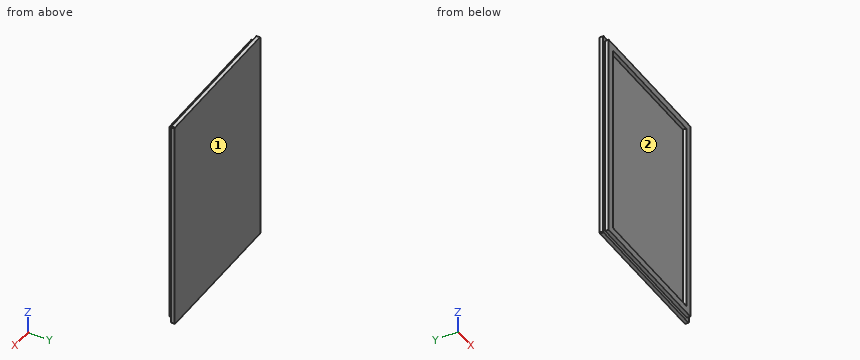
Autodesk Inventor part; units mm, degrees
ref_plane "YZ Plane" through (0, 0, 0) normal (1, 0, 0) x (0, 1, 0)
ref_plane "XZ Plane" through (0, 0, 0) normal (0, 1, 0) x (-1, 0, 0)
ref_plane "XY Plane" through (0, 0, 0) normal (0, 0, 1) x (1, 0, 0)
sketch "Sketch1" plane through (0, 0, 0) normal (0, 1, 0) x (-1, 0, 0)
  line L0 (0, 0) -> (210, 0)
  line L1 (210, 0) -> (210, -310)
  line L2 (210, -310) -> (0, -310)
  line L3 (0, -310) -> (0, 0)
  dimension "d0" = 310
  dimension "d1" = 210
extrude "Extrusion1" add sketch "Sketch1" along normal blind 5
chamfer "Chamfer1" distance 1 angle 45 4 edges at (0, 2.5, -310) (0, 2.5, 0) (-210, 2.5, -310) (-210, 2.5, 0)
sketch "Sketch2" plane through (0, 0, 0) normal (0, -1, 0) x (1, 0, 0)
  line L0 (-205, -305) -> (-5, -305)
  line L1 (-5, -305) -> (-5, -5)
  line L2 (-5, -5) -> (-205, -5)
  line L3 (-205, -5) -> (-205, -305)
  line L4 (0, -1) -> (0, -309)
  line L5 (-209, 0) -> (-1, 0)
  point P0 (0, 0)
  dimension "d7" = 300
  dimension "d8" = 200
  dimension "d9" = 5
  dimension "d10" = 5
extrude "Extrusion2" add sketch "Sketch2" along normal blind 5
sketch "Sketch3" plane through (0, -5, 0) normal (0, -1, 0) x (1, 0, 0)
  line L0 (-195, -295) -> (-15, -295)
  line L1 (-15, -295) -> (-15, -15)
  line L2 (-15, -15) -> (-195, -15)
  line L3 (-195, -15) -> (-195, -295)
  line L4 (-5, -5) -> (-205, -5)
  line L5 (-205, -5) -> (-205, -305)
  point P0 (0, 0)
  dimension "d13" = 280
  dimension "d14" = 180
  dimension "d15" = 10
  dimension "d16" = 10
extrude "Extrusion3" cut sketch "Sketch3" against normal blind 5
properties part number "Tutup_Box"
The listing builds one solid part. Answer for the finished solid, in the listing's coordinates (mm). Face numbers are marked on the shaded views. Give positions to 0.01 mm unless a question says otherwise; leave off trailing zeros. Write each loop counter-clockwise with the first axis right and the second up, starting at its lowest first coordinate (ties: lowest second). Pieces come first, ordered by that corner, then holes. Notation, with made-up numbers: (38.5, -35.75) -> (93.5, -35.75) arc R18 cw to (93.5, -4.75) -> close; hole circle Ø8 at (47, 74.25). An arc over 180 degrees is marked (long way). Use a Markdown table: item, result.
(1) Flat-ended cylindrical pins translate along their axes: P1, Ø1.5, axis at y = -3, z = -123, coming from the +X side; P2, Ø4, axis at y = -3.5, z = -111, coming from the -X side; P3, Ø4, axis at x = -74, z = -165.5, coming from the -Y side. Find the tip coordinate at first contact, or state that the pin passes through.
Return value:
| item | result |
|---|---|
| P1 | x = -5 |
| P2 | x = -205 |
| P3 | y = 0 |
(2) Determine the mould class of the marked faces 1 and 2 for opening direction X: released by +X, released by -X, zero draft, split by the parting line, or undercut.
Return value:
| item | result |
|---|---|
| face 1 | zero draft |
| face 2 | undercut |
(3) Find the intervals of material crossed by probe 1 along Z at (x, y) = (-72.5, -3); probe 2 along X at (y, z) = (-1.5, -157); probe 3 along Y at (x, z) = (-47, -187), in increasing order. Write a range as from..to.
Return value:
| item | result |
|---|---|
| probe 1 | -305..-295, -15..-5 |
| probe 2 | -205..-195, -15..-5 |
| probe 3 | 0..5 |
(4) Section C-C, the plane z = -124 is taken. Determine the outline of the cut face in (x, y), then the cut area to 3 significant figures.
Return value:
| item | result |
|---|---|
| outline | (-210, 0) -> (-205, 0) -> (-205, -5) -> (-195, -5) -> (-195, 0) -> (-15, 0) -> (-15, -5) -> (-5, -5) -> (-5, 0) -> (0, 0) -> (0, 5) -> (-210, 5) -> close |
| area | 1,150 mm2 |
(5) Section B-B, the plane x = -178 is taken. Determine the outline of the cut face in (y, z).
Return value:
| item | result |
|---|---|
| outline | (-5, -305) -> (0, -305) -> (0, -310) -> (5, -310) -> (5, 0) -> (0, 0) -> (0, -5) -> (-5, -5) -> (-5, -15) -> (0, -15) -> (0, -295) -> (-5, -295) -> close |
(6) Section A-A, the plane y = -3.25 is taken. Determine the outline of the cut face in (x, z).
Return value:
| item | result |
|---|---|
| outline | (-205, -305) -> (-5, -305) -> (-5, -5) -> (-205, -5) -> close; hole (-195, -295) -> (-15, -295) -> (-15, -15) -> (-195, -15) -> close |
